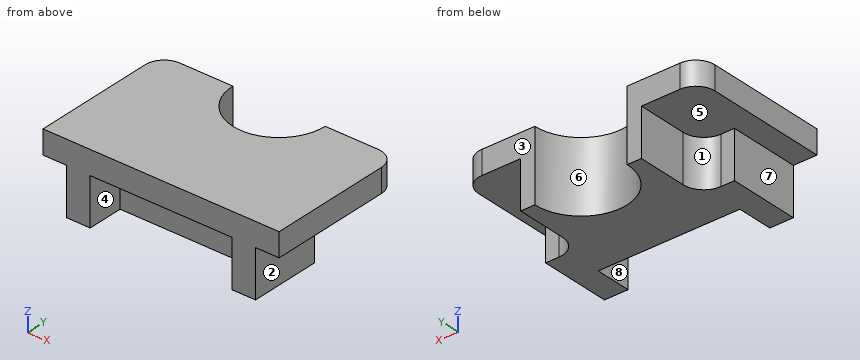
```python
from build123d import *

# Parameters (mm, degrees)
F1_DEPTH = 6.35
F3_DEPTH = 12.7
F4_R     = 5.538906
F5_R     = 5.08


with BuildPart() as f1:
    # F0 (on Top) → F1 (new body)
    with BuildSketch(Plane.XY):
        with BuildLine():
            Line((-12.4206, 19.05), (-31.75, 19.05))
            Line((-31.75, 19.05), (-31.75, -19.05))
            Line((-31.75, -19.05), (31.75, -19.05))
            Line((31.75, -19.05), (31.75, 19.05))
            Line((31.75, 19.05), (12.4206, 19.05))
            ThreePointArc((12.4206, 19.05), (0, 6.6294), (-12.4206, 19.05))
        make_face()
    extrude(amount=F1_DEPTH)

    # F2 (on Top) → F3 (join)
    with BuildSketch(Plane.XY):
        with BuildLine():
            Line((-12.4206, 19.05), (-16.2306, 19.05))
            Line((-16.2306, 19.05), (-16.2306, 0))
            Line((-16.2306, 0), (-25.4, 0))
            Line((-25.4, 0), (-25.4, -19.05))
            Line((-25.4, -19.05), (-19.05, -19.05))
            Line((-19.05, -19.05), (-19.05, -9.398))
            Line((-19.05, -9.398), (19.05, -9.398))
            Line((19.05, -9.398), (19.05, -19.05))
            Line((19.05, -19.05), (25.4, -19.05))
            Line((25.4, -19.05), (25.4, 0))
            Line((25.4, 0), (16.2306, 0))
            Line((16.2306, 0), (16.2306, 19.05))
            Line((16.2306, 19.05), (12.4206, 19.05))
            ThreePointArc((12.4206, 19.05), (0, 6.6294), (-12.4206, 19.05))
        make_face()
    extrude(amount=-F3_DEPTH)

    # F4
    f4_edges = [f1.edges().sort_by_distance(p)[0] for p in [
        (16.2306, 0, -6.35),
        (-16.2306, 0, -6.35),
    ]]
    fillet(f4_edges, radius=F4_R)

    # F5
    f5_edges = [f1.edges().sort_by_distance(p)[0] for p in [
        (31.75, 19.05, 3.175),
        (-31.75, 19.05, 3.175),
    ]]
    fillet(f5_edges, radius=F5_R)


solid = f1.part
```
The model under review builds one solid part; all positions refer to its coordinate system, in mm. Face numbers are marked on the shaded views. A direction names the side the tool comes from. Round coordinates to 2 decimals unless told otherwise and drop trailing zeros. Loops run counter-clockwise (first coordinate to the right, second up) from the corner with the lowest first, then second, coordinate; pieces in that order, holes last. Notation, with made-up numbers: M 54,29 L 60,29 A28 ccw 60,68 Z; hole C 67.5,1.5 d10. An arc over 180 degrees is marked long. Write item = value, one per line.
Item 1: Take a section at C-C on x = 0. Write out the cut boundary in (y, z), then the cut area to 3 significant figures.
Return value:
outline = M -19.05,0 L -9.4,0 L -9.4,-12.7 L 6.63,-12.7 L 6.63,6.35 L -19.05,6.35 Z
area = 367 mm2
Item 2: Take a section at A-A on z = -9.25. Write out the cut boundary in (x, y), then the cut area to 3 significant figures.
Return value:
outline = M -25.4,-19.05 L -19.05,-19.05 L -19.05,-9.4 L 19.05,-9.4 L 19.05,-19.05 L 25.4,-19.05 L 25.4,0 L 21.77,0 A5.54 cw 16.23,5.54 L 16.23,19.05 L 12.42,19.05 A12.42 cw -12.42,19.05 L -16.23,19.05 L -16.23,5.54 A5.54 cw -21.77,0 L -25.4,0 Z
area = 989 mm2
Item 3: Insertion check: P1, Ø3, axis at x = -24, z = -9, coming from the +Y side; P2, Ø10.5, axis at x = -7, y = -16.5, coming from the -Z side; P3, Ø6.5, axis at y = -12, z = -7, coming from the -X side. Each pin has a flat end and moves straight along its axis. Give the tip position at first contact, or say it passes through.
Return value:
P1 = 0
P2 = 0
P3 = -25.4
Item 4: Take a section at B-B on y = -7.5. Write out the cut boundary in (x, z), then the cut area to 3 significant figures.
Return value:
outline = M -31.75,0 L -25.4,0 L -25.4,-12.7 L 25.4,-12.7 L 25.4,0 L 31.75,0 L 31.75,6.35 L -31.75,6.35 Z
area = 1,050 mm2
Item 5: For line 1 (X direction, y = -14, z = -0.25); line 2 (Z direction, x = -27, y = -9.5); line 3 (Y direction, x = 16, z = -7), list the stretches that pass through material, from the lowest coordinate up. Write a range as [from, to].
Return value:
line_1 = [-25.4, -19.05], [19.05, 25.4]
line_2 = [0, 6.35]
line_3 = [-9.4, 19.05]
Item 6: The part is to be moulded in two halves that separate along X. For the marked faces 5, 6, 7 and 8, say which applies: released by +X, released by -X, zero draft, split by the parting line, or undercut.
Return value:
face_5 = zero draft
face_6 = undercut
face_7 = released by -X
face_8 = undercut
Item 7: Take a section at D-D on z = 3. Write out the cut boundary in (x, y), then the cut area to 3 significant figures.
Return value:
outline = M -31.75,-19.05 L 31.75,-19.05 L 31.75,13.97 A5.08 ccw 26.67,19.05 L 12.42,19.05 A12.42 cw -12.42,19.05 L -26.67,19.05 A5.08 ccw -31.75,13.97 Z
area = 2,170 mm2
Item 8: Machinability: for the marked faces 1, 2, 3 and 4, which of the approach directions +Z, -Z, +X, -X, +Y, -Y give a long, thin tool a straight path to every point of the face, cutting with its end or side? Answer none if there is none.
Return value:
face_1 = -Z, -X, +Y
face_2 = -Z, +X, +Y, -Y
face_3 = +Z, -Z, +X, -X, +Y
face_4 = -Z, -Y
